Geometry check sheet. Reference: drawing and pictorial views, mm from the part's lowest x, y, z. A direction names the side the tool comes from. Give positions to 0.01 mm unless a question says otherwise; leave off trailing zeros. Order: outer loops, then holes, each group sorted by start corner. A loop starts at its lowest first (then second) coordinate and runs counter-clockwise, first axis right, second up.
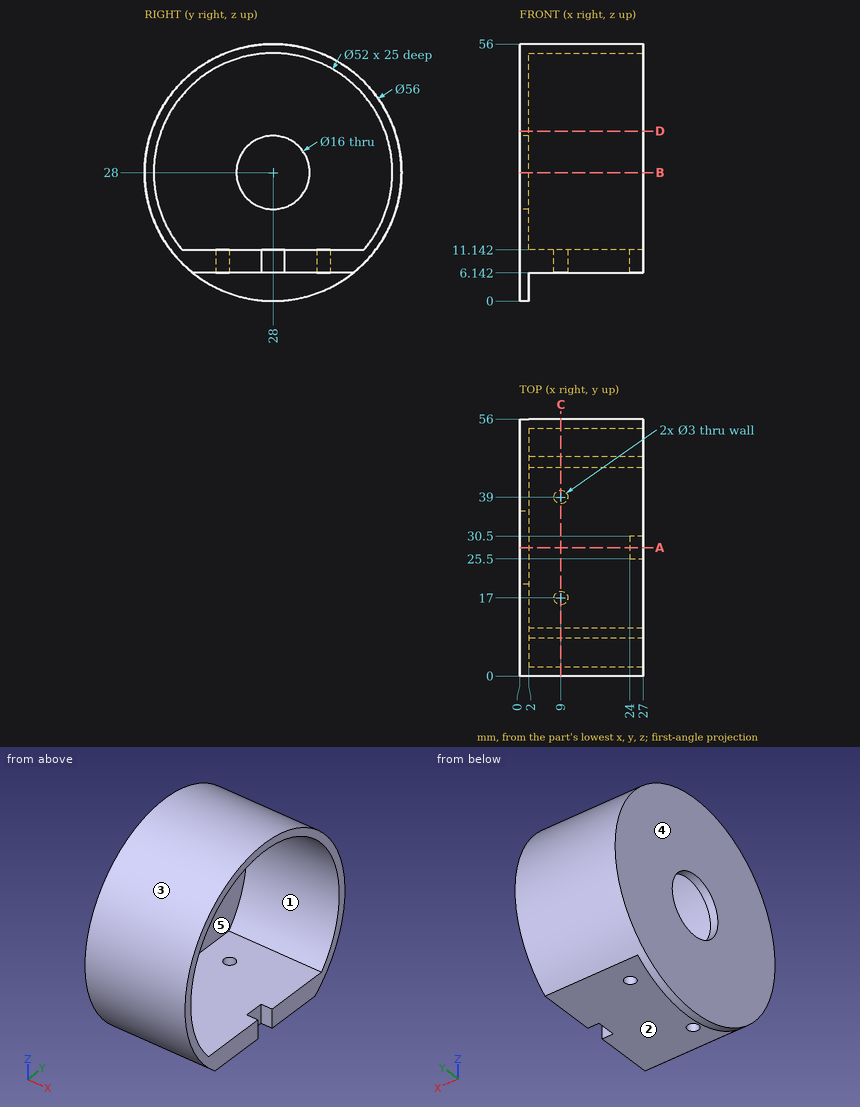
1) Section check A-A, the plane y = 28. Record the cut outline in (x, z).
Recorded:
outline: (0, 0) - (2, 0) - (2, 6.14) - (24, 6.14) - (24, 11.14) - (2, 11.14) - (2, 20) - (0, 20) - close; (0, 36) - (2, 36) - (2, 54) - (27, 54) - (27, 56) - (0, 56) - close
2) Set-up check for the marked faces 4 and 5: record each of +Z, -Z, +X, -X, +Y, -Y from which the full face is reachable in a straight line by a thin tool's end or side.
Recorded:
face 4: +Z, -Z, -X, +Y, -Y
face 5: +X
3) Depth check by flat-ended pin: pin 1 Ø6 at (y, z) = (16.5, 41) entering from +X; pin 2 Ø3.5 at (x, y) = (9, 17) entering from +Z; pin 3 Ø2.5 at (x, y) = (9, 39) entering from -Z. Enter the tip coordinate at first touch or a pass-through.
Recorded:
pin 1: stops at x = 2
pin 2: stops at z = 54.43
pin 3: stops at z = 50.93
4) Material ranges on L1, parallel to Z at x = 9.25, y = 28; L2, parallel to Y at x = 9, z = 9 (1 decimal); L3, parallel to Z at x = 0.85, y = 28, recorded low to high.
Recorded:
L1: z = 6.14 to 11.14, 54 to 56
L2: y = 7.4 to 15.5, 18.5 to 37.5, 40.5 to 48.6
L3: z = 0 to 20, 36 to 56
5) Draft check along Z on the marked faces 1, 2 and 3. Enter one of: +Z half, -Z half, draft (parallel to the pull), parting line (faces both ways), or undercut.
Recorded:
face 1: undercut
face 2: -Z half
face 3: parting line
6) Section check B-B, the plane z = 28. Record the cut outline in (x, y), then the cut area to 3 significant figures.
Recorded:
outline: (0, 0) - (27, 0) - (27, 2) - (2, 2) - (2, 20) - (0, 20) - close; (0, 36) - (2, 36) - (2, 54) - (27, 54) - (27, 56) - (0, 56) - close
area: 180 mm2
7) Section check D-D, the plane z = 37. Record the cut outline in (x, y) (1 decimal), then the cut area to 3 significant figures.
Recorded:
outline: (0, 1.5) - (27, 1.5) - (27, 3.6) - (2, 3.6) - (2, 52.4) - (27, 52.4) - (27, 54.5) - (0, 54.5) - close
area: 212 mm2
8) Section check C-C, the plane x = 9. Record the cut outline in (y, z) (1 decimal).
Recorded:
outline: (8.2, 11.1) arc R26 cw (long way) to (47.8, 11.1) - (40.5, 11.1) - (40.5, 6.1) - (45.5, 6.1) arc R28 ccw (long way) to (10.5, 6.1) - (15.5, 6.1) - (15.5, 11.1) - close; (18.5, 6.1) - (37.5, 6.1) - (37.5, 11.1) - (18.5, 11.1) - close
